Can you work these out from the model? Positions are in its coordinate system, mm. Coordinates: 2 decimals unless noted, no trailing zeros. Loops run counter-clockwise (first coordinate to the right, second up) from the corner with the lowest first, then second, coordinate; pieces in that order, holes last.
```python
from build123d import *

# Parameters (mm, degrees)
SKETCH1_R           = 4
BOSS_EXTRUDE1_DEPTH = 2
CHAMFER1_SIZE       = 0.5


with BuildPart() as part:
    # Sketch1 → Boss-Extrude1 (new body)
    with BuildSketch(Plane.XY):
        Polygon((2.886751346, 5), (-2.886751346, 5), (-5.773502692, 0), (-2.886751346, -5), (2.886751346, -5), (5.773502692, 0), align=None)
        Circle(SKETCH1_R, mode=Mode.SUBTRACT)
    extrude(amount=BOSS_EXTRUDE1_DEPTH)

    # Chamfer1
    chamfer1_edges = [part.edges().sort_by_distance(p)[0] for p in [
        (-4.330127019, 2.5, 2),
        (-4.330127019, -2.5, 2),
        (0, -5, 2),
        (4.330127019, -2.5, 2),
        (4.330127019, 2.5, 2),
        (4.330127019, -2.5, 0),
        (0, -5, 0),
        (-4.330127019, -2.5, 0),
        (-4.330127019, 2.5, 0),
        (0, 5, 0),
        (4.330127019, 2.5, 0),
        (0, 5, 2),
    ]]
    chamfer(chamfer1_edges, length=CHAMFER1_SIZE)


solid = part.part
```
Item 1: I need wall thicknesses on line 1 along Y through (x, z) = (0, 0.75); line 2 along X through (y, z) = (3, 0.3); line 3 along X through (y, z) = (-1.25, 1.6). Which ranges of each line are inside material? Lowest first, please.
Results are:
line 1: y = -5 to -4, 4 to 5
line 2: x = -3.81 to -2.65, 2.65 to 3.81
line 3: x = -4.94 to -3.8, 3.8 to 4.94
Item 2: Suppose I cut it at B-B, the plane y = -0.5. Please give me the cut outline in (x, z), plus the area to 3 significant figures.
Results are:
outline: (-5.48, 0.5) - (-4.91, 0) - (-3.97, 0) - (-3.97, 2) - (-4.91, 2) - (-5.48, 1.5) - close; (3.97, 0) - (4.91, 0) - (5.48, 0.5) - (5.48, 1.5) - (4.91, 2) - (3.97, 2) - close
area: 5.49 mm2
Item 3: Suppose I cut it at C-C, the plane x = 0. Please give me the cut outline in (y, z), plus the area to 3 significant figures.
Results are:
outline: (-5, 0.5) - (-4.5, 0) - (-4, 0) - (-4, 2) - (-4.5, 2) - (-5, 1.5) - close; (4, 0) - (4.5, 0) - (5, 0.5) - (5, 1.5) - (4.5, 2) - (4, 2) - close
area: 3.50 mm2
Item 4: I'm going to push a flat-ended pin straight in: P1, Ø2, axis at x = 2.5, y = 2, coming from the -Z side. Where does the tip first touch, or does it pass through?
Results are:
P1: stops at z = 0
Item 5: We'd pull the mould along X, two halves only. Please class faces 1 (the face through (0, 5, 1)), 2 (the face through (4.09, -2.408, 1.754)), 3 (the face through (-0.867, -3.905, 0.986)), 4 (the face through (-4.35, -2.465, 0.993)): +X half, -X half, draft (parallel to the pull), parting line (faces both ways), or undercut.
Results are:
face 1: draft
face 2: +X half
face 3: undercut
face 4: -X half
Item 6: Suppose I cut it at D-D, the plane z = 1.8. Please give me the cut outline in (x, y).
Results are:
outline: (-5.43, 0) - (-2.71, -4.7) - (2.71, -4.7) - (5.43, 0) - (2.71, 4.7) - (-2.71, 4.7) - close; hole circle Ø8 at (0, 0)
Item 7: Suppose I cut it at A-A, the plane z = 0.8. Please give me the cut outline in (x, y), plus the area to 3 significant figures.
Results are:
outline: (-5.77, 0) - (-2.89, -5) - (2.89, -5) - (5.77, 0) - (2.89, 5) - (-2.89, 5) - close; hole circle Ø8 at (0, 0)
area: 36.3 mm2
